Job drawing, mm, ordinate dimensions from the low corner. One solid piece. A direction names the side the tool comes from. Give positions to 0.01 mm unless a question says otherwise; leave off trailing zeros. Order: outer loops, then holes, each group sorted by start corner. A loop starts at its lowest first (then second) coordinate and runs counter-clockwise, first axis right, second up. Notation, with made-up numbers: (71, 54) -> (89, 54) arc R20 ccw to (89, 81) -> close; hole circle Ø11 at (-30, -32.5). An arc over 180 degrees is marked (long way). Write item = value, one per line. Start each with the question number.
(1) Probe line 1 along Z through (x, y) = (5.5, 16.5); line 2 along Y through (x, z) = (2, 16.5); line 3 along Y through (x, z) = (1.5, 19). List the from-to ranges inside material, lowest first. Write a range as from..to.
(2) Saw through at B-B, the plane y = 16.5. List the corners of the cut face in (x, z), then the cut area to 3 significant figures.
(3) Saw through at C-C, the plane x = 2.75. List the corners of the cut face in (y, z), then the cut area to 3 significant figures.
(4) Saw through at A-A, the plane z = 16.5. List the corners of the cut face in (x, y), then the cut area to 3 significant figures.
(5) Saw through at D-D, the plane x = 6. List the corners of the cut face in (y, z), then the cut area to 3 significant figures.
(6) Flat gauge pins, fed straight in: pin 1 (1.5 mm diameter, centred on x = 5, y = 18, fed in from -Z); pin 2 (2 mm diameter, centred on y = 9.5, z = 13.5, fed in from +X); pin 3 (1.3 mm diameter, centred on x = 2.5, z = 19, fed in from -Y); pin 4 (0.6 mm diameter, centred on x = 2.5, y = 7, fed in from -Z). Where does each tip first touch, or does it go through?
(7) Two-plate mould, pull along Z, no slides. Class the marked faces 1, 2 and 3: pulls with the +Z half, pulls with the -Z half, needs draft (parallel to the pull), parting line crosses it, or undercut.
(8) Which spindle directions (+Z, -Z, +X, -X, +Y, -Y) get a long thin tool onto all of the face, cutting with end or side? Do the marked faces 4 and 5. Say none if no direction does.
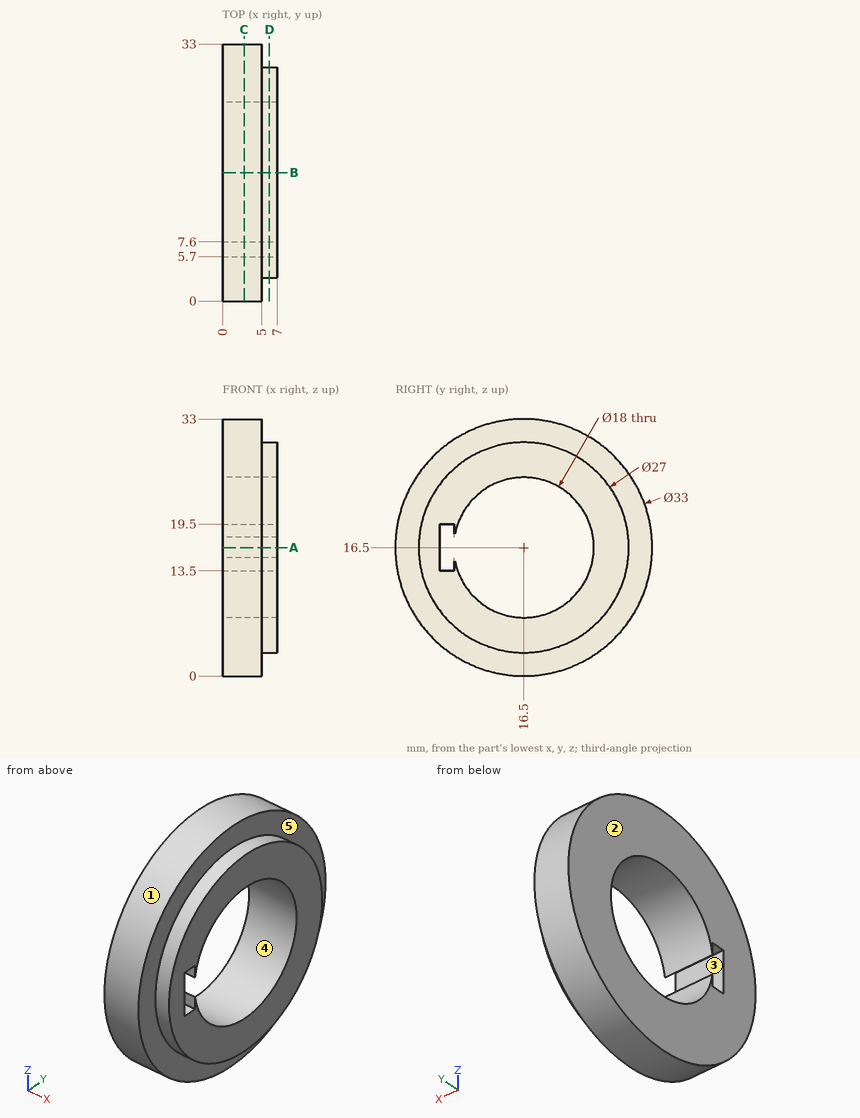
Results list:
q1.line_1 = 3..7.5, 25.5..30
q1.line_2 = 0..5.7, 25.5..33
q1.line_3 = 0.19..5.7, 7.6..7.85, 25.15..32.81
q2.outline = (0, 0) -> (5, 0) -> (5, 3) -> (7, 3) -> (7, 7.5) -> (0, 7.5) -> close; (0, 25.5) -> (7, 25.5) -> (7, 30) -> (5, 30) -> (5, 33) -> (0, 33) -> close
q2.area = 93.0 mm^2
q3.outline = circle Ø33 at (16.5, 16.5); hole (5.7, 13.5) -> (7.6, 13.5) -> (7.6, 15.16) arc R9 ccw (long way) to (7.6, 17.84) -> (7.6, 19.5) -> (5.7, 19.5) -> close
q3.area = 590 mm^2
q4.outline = (0, 0) -> (5, 0) -> (5, 3) -> (7, 3) -> (7, 5.7) -> (0, 5.7) -> close; (0, 25.5) -> (7, 25.5) -> (7, 30) -> (5, 30) -> (5, 33) -> (0, 33) -> close
q4.area = 80.4 mm^2
q5.outline = circle Ø27 at (16.5, 16.5); hole (5.7, 13.5) -> (7.6, 13.5) -> (7.6, 15.16) arc R9 ccw (long way) to (7.6, 17.84) -> (7.6, 19.5) -> (5.7, 19.5) -> close
q5.area = 307 mm^2
q6.pin_1 = 0.02
q6.pin_2 = through
q6.pin_3 = 0.1
q6.pin_4 = 2.8
q7.face_1 = parting line crosses it
q7.face_2 = needs draft
q7.face_3 = undercut
q8.face_4 = +X, -X
q8.face_5 = +X
